Check sheet for the modelled part. Datum: model origin and axes. Units: mm. A direction names the side the tool comes from. Give positions to 0.01 mm unless a question says otherwise; leave off trailing zeros. Write each loop counter-clockwise with the first axis right and the second up, starting at its lowest first coordinate (ties: lowest second). Pieces come first, ordered by that corner, then holes. Notation, with made-up numbers: (53, -25) -> (98, -25) arc R22 cw to (98, 3) -> close; hole circle Ø3 at (-2, 60.5). An arc over 180 degrees is marked (long way). Use a Markdown table: item, result. Add a question column.
1. Cross-section at C-C (y = 89.5). Enter the section's corners in (x, z).
2. Gauge pin test, flat ends, axial feed: P1, Ø4, axis at y = 53.5, z = 48, coming from the -X side; P2, Ø9.5, axis at x = 36.16, y = 80, coming from the +Z side; P3, Ø4, axis at x = -30, y = 33.5, coming from the +Z side; P4, Ø2.5, axis at x = 36.16, y = 40, coming from the -Z side. Record the tip position at first contact, or that the pin passes through.
3. Scan lines: probe 1 along X at (y, z) = (80, 28.8); probe 2 along Y at (x, z) = (37, 34.5); probe 3 along X at (y, z) = (40, 35.25). Record each from-to range of solid material in increasing order. Write a range as [from, to].
4. Cross-section at B-B (x = 2). Enter the section's corners in (y, z).
5. Set-up check for faces 5 (the cylindrical face through (33.267, 20.128, 33.428)), 6 (the cylindrical face through (33.267, 80.128, 33.427)), 7 (the cylindrical face through (-0.695, 6.542, 50.287)): record each of +Z, -Z, +X, -X, +Y, -Y from which the full face is reachable in a straight line by a thin tool's end or side.
6. Cross-section at A-A (y = 40). Enter the section's corners in (x, z).
7. Release check for a two-part mould opening along Z. For faces 1 (the conical face through (-38, 19, 30)), 2 (the conical face through (-38, 59, 30)), 3 (the flat face through (-0.6, 0, 41.3)), 4 (the cylindrical face through (-33.267, 20.128, 33.428)) record: released by +Z, released by -Z, zero draft, split by the parting line, or undercut.
8. Cross-section at D-D (x = -23). Enter the section's corners in (y, z).
from build123d import *

# Parameters (mm, degrees)
BOSS_EXTRUDE1_DEPTH      = 100
LPATTERN1_COUNT          = 4
LPATTERN1_PITCH          = 20
BOSS_EXTRUDE2_DEPTH      = 6.731
BOSS_EXTRUDE2_DEPTH_BACK = 6.731
SKETCH9_R                = 3.334469726
CUT_EXTRUDE1_DEPTH       = 34
BOSS_EXTRUDE3_DEPTH      = 40


with BuildPart() as part:
    # Sketch1 → Boss-Extrude1 (new body)
    with BuildSketch(Plane(origin=(60.535204745, 0, -85.948449604), x_dir=(1, 0, 0), z_dir=(0, 1, 0))):
        with BuildLine():
            ThreePointArc((-30.186446753, -113.644462538), (-60.535204745, -127.035141416), (-90.883962736, -113.644462538))
            Line((-90.883962736, -113.644462538), (-102.513962844, -113.644462538))
            ThreePointArc((-102.513962844, -113.644462538), (-60.535204745, -136.240449604), (-18.556446645, -113.644462538))
            Line((-18.556446645, -113.644462538), (-30.186446753, -113.644462538))
        make_face()
    extrude(amount=BOSS_EXTRUDE1_DEPTH)

    # Sketch6 → Cut-Revolve4 (revolve, cut)
    with BuildSketch(Plane(origin=(36.163758045, 20, 27.696012934), x_dir=(-1, 0, 0), z_dir=(0, -1, 0))):
        Polygon((0, 1.685394277), (0, -4.78184701), (0, -15.185924704), (-2.9, -15.185924704), (-2.9, -3.079025683), (-1.65, -1.881964943), (-1.65, 1.685394277), align=None)
    cut_revolve4 = revolve(axis=Axis((36.163758045, 20, 26.010618657), (0, 0, 1)), mode=Mode.SUBTRACT)

    # LPattern1: Cut-Revolve4 ×4
    with Locations(*[(0, i * LPATTERN1_PITCH, 0) for i in range(1, LPATTERN1_COUNT)]):
        add(cut_revolve4, mode=Mode.SUBTRACT)

    # Mirror1: Cut-Revolve4 across plane
    add(cut_revolve4.mirror(Plane(origin=(0, 0, 0), x_dir=(0, 0, 1), z_dir=(1, 0, 0))), mode=Mode.SUBTRACT)

    # Mirror1 copy 1 sketch → Mirror1 copy 1 (revolve, cut)
    with BuildSketch(Plane(origin=(-36.163758045, 40, 27.696012934), x_dir=(1, 0, 0), z_dir=(0, -1, 0))):
        Polygon((0, -1.685394277), (0, 4.78184701), (0, 15.185924704), (-2.9, 15.185924704), (-2.9, 3.079025683), (-1.65, 1.881964943), (-1.65, -1.685394277), align=None)
    revolve(axis=Axis((-36.163758045, 40, 26.010618657), (0, 0, -1)), mode=Mode.SUBTRACT)

    # Mirror1 copy 2 sketch → Mirror1 copy 2 (revolve, cut)
    with BuildSketch(Plane(origin=(-36.163758045, 60, 27.696012934), x_dir=(1, 0, 0), z_dir=(0, -1, 0))):
        Polygon((0, -1.685394277), (0, 4.78184701), (0, 15.185924704), (-2.9, 15.185924704), (-2.9, 3.079025683), (-1.65, 1.881964943), (-1.65, -1.685394277), align=None)
    revolve(axis=Axis((-36.163758045, 60, 26.010618657), (0, 0, -1)), mode=Mode.SUBTRACT)

    # Mirror1 copy 3 sketch → Mirror1 copy 3 (revolve, cut)
    with BuildSketch(Plane(origin=(-36.163758045, 80, 27.696012934), x_dir=(1, 0, 0), z_dir=(0, -1, 0))):
        Polygon((0, -1.685394277), (0, 4.78184701), (0, 15.185924704), (-2.9, 15.185924704), (-2.9, 3.079025683), (-1.65, 1.881964943), (-1.65, -1.685394277), align=None)
    revolve(axis=Axis((-36.163758045, 80, 26.010618657), (0, 0, -1)), mode=Mode.SUBTRACT)

    # Sketch7 → Boss-Extrude2 (add, two sides)
    with BuildSketch(Plane(origin=(0, 20, 0), x_dir=(-1, 0, 0), z_dir=(0, -1, 0))) as boss_extrude2_sk:
        with BuildLine():
            Line((-44.990566695, -27.696012934), (-41.978758099, -27.696012934))
            ThreePointArc((-41.978758099, -27.696012934), (0, -50.292), (41.978758099, -27.696012934))
            Line((41.978758099, -27.696012934), (44.990566695, -27.696012934))
            ThreePointArc((44.990566695, -27.696012934), (0, -52.832), (-44.990566695, -27.696012934))
        make_face()
    extrude(amount=BOSS_EXTRUDE2_DEPTH)
    extrude(boss_extrude2_sk.sketch, amount=-BOSS_EXTRUDE2_DEPTH_BACK)

    # Sketch9 → Cut-Extrude1 (cut)
    with BuildSketch(Plane(origin=(0, 0, 27.696012934), x_dir=(-1, 0, 0), z_dir=(0, 0, -1))):
        with Locations((-18.801989508, 20)):
            Circle(SKETCH9_R)
        with Locations((-8.69556827, 20)):
            Circle(SKETCH9_R)
    extrude(amount=-CUT_EXTRUDE1_DEPTH, mode=Mode.SUBTRACT)

    # Sketch10 → Boss-Extrude3 (add)
    with BuildSketch(Plane(origin=(0, 100, 0), x_dir=(1, 0, 0), z_dir=(0, 1, 0))):
        with BuildLine():
            Line((-30.348757991, -27.696012934), (-41.978758099, -27.696012934))
            ThreePointArc((-41.978758099, -27.696012934), (0, -50.292), (41.978758099, -27.696012934))
            Line((41.978758099, -27.696012934), (30.348757991, -27.696012934))
            ThreePointArc((30.348757991, -27.696012934), (0, -41.086691812), (-30.348757991, -27.696012934))
        make_face()
    extrude(amount=BOSS_EXTRUDE3_DEPTH)


solid = part.part
Worked answers:
| question | item | result |
|---|---|---|
| 1 | outline | (-41.98, 27.7) -> (-30.35, 27.7) arc R41.09 cw to (30.35, 27.7) -> (41.98, 27.7) arc R50.29 ccw to start |
| 2 | P1 | stops at x = -20.33 |
| 2 | P2 | stops at z = 39.28 |
| 2 | P3 | stops at z = 41.78 |
| 2 | P4 | passes through |
| 3 | probe 1 | x = [-41.23, -37.81], [-34.51, -29.3], [29.3, 34.51], [37.81, 41.23] |
| 3 | probe 2 | y = [13.27, 26.73] |
| 3 | probe 3 | x = [-33.26, -21.11], [21.11, 33.26] |
| 4 | outline | (0, 41.04) -> (140, 41.04) -> (140, 50.25) -> (26.73, 50.25) -> (26.73, 52.79) -> (13.27, 52.79) -> (13.27, 50.25) -> (0, 50.25) -> close |
| 5 | face 5 | none |
| 5 | face 6 | +Z |
| 5 | face 7 | +Z, -Y |
| 6 | outline | (-41.98, 27.7) -> (-37.81, 27.7) -> (-37.81, 29.58) -> (-39.06, 30.78) -> (-39.06, 31.68) arc R50.29 ccw to start; (-34.51, 27.7) -> (-30.35, 27.7) arc R41.09 cw to (30.35, 27.7) -> (34.51, 27.7) -> (34.51, 29.58) -> (33.26, 30.78) -> (33.26, 37.72) arc R50.29 ccw to (-33.26, 37.72) -> (-33.26, 30.78) -> (-34.51, 29.58) -> close; (37.81, 27.7) -> (41.98, 27.7) arc R50.29 ccw to (39.06, 31.68) -> (39.06, 30.78) -> (37.81, 29.58) -> close |
| 7 | face 1 | undercut |
| 7 | face 2 | released by +Z |
| 7 | face 3 | zero draft |
| 7 | face 4 | undercut |
| 8 | outline | (0, 34.05) -> (140, 34.05) -> (140, 44.72) -> (26.73, 44.72) -> (26.73, 47.56) -> (13.27, 47.56) -> (13.27, 44.72) -> (0, 44.72) -> close |
